from build123d import *

# Parameters (mm, degrees)
EXTRUDE_1_DEPTH     = 16
SKETCH_2_R          = 2.5
CUT_EXTRUDE_1_DEPTH = 9
SKETCH_3_R          = 4
CUT_EXTRUDE_2_DEPTH = 29


with BuildPart() as part:
    # 草图1 → 凸台-拉伸1 (new body)
    with BuildSketch(Plane.XY):
        Polygon((0, 0), (16, 0), (16, 8), (8, 8), (8, 40), (-8, 40), (-8, 8), (-16, 8), (-16, 0), align=None)
    extrude(amount=EXTRUDE_1_DEPTH)

    # 草图2 → 切除-拉伸1 (cut, through all)
    with BuildSketch(Plane(origin=(0, 8, 0), x_dir=(1, 0, 0), z_dir=(0, 1, 0))):
        with Locations((-12, -8)):
            Circle(SKETCH_2_R)
        with Locations((12, -8)):
            Circle(SKETCH_2_R)
    extrude(amount=-CUT_EXTRUDE_1_DEPTH, mode=Mode.SUBTRACT)

    # 草图3 → 切除-拉伸2 (cut)
    with BuildSketch(Plane.XY.offset(16)):
        with Locations((0, 31.77)):
            Circle(SKETCH_3_R)
    extrude(amount=-CUT_EXTRUDE_2_DEPTH, mode=Mode.SUBTRACT)


solid = part.part
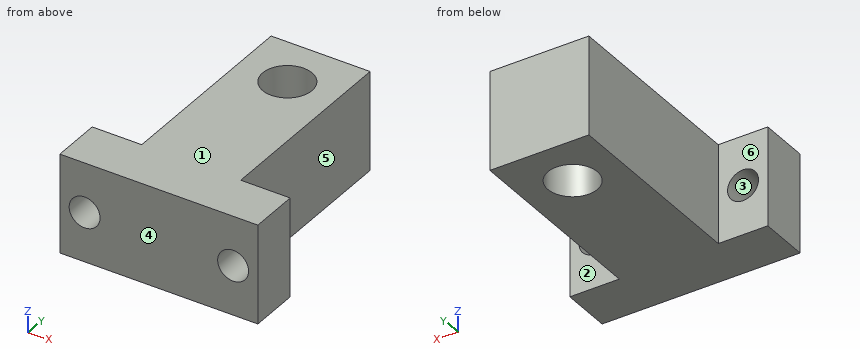
Geometry check sheet. Reference: the model listing, model coordinates, mm. Face numbers are marked on the shaded views. A direction names the side the tool comes from. Round coordinates to 2 decimals unless told otherwise and drop trailing zeros. Order: outer loops, then holes, each group sorted by start corner. A loop starts at its lowest first (then second) coordinate and runs counter-clockwise, first axis right, second up. Notation, with made-up numbers: M -14.75,-35 L 35.25,-35 A24 ccw 35.25,-10 Z; hole C 12,-8.5 d2. An arc over 180 degrees is marked long. Write each question's results on one line, items separated by ' | '. Start each with the question number.
1. Cross-section at D-D on z = 1. Record the boundary of the cut face in (x, y).
2. Set-up check for the marked faces 4, 5 and 6: record each of +Z, -Z, +X, -X, +Y, -Y from which the full face is reachable in a straight line by a thin tool's end or side.
3. Cross-section at A-A on z = 8. Record the boundary of the cut face in (x, y).
4. Material ranges on L1, parallel to X at y = 2.25, z = 8; L2, parallel to Y at x = 0, z = 5; L3, parallel to Z at x = -12, y = 3, recorded low to high. Write a range as from..to.
5. Cross-section at B-B on y = 31.77. Record the boundary of the cut face in (x, z), plus the area to 3 significant figures.
6. Cross-section at C-C on x = 0. Record the boundary of the cut face in (y, z).
7. Go/stop test with flat-tipped pins: P1, Ø6.5, axis at x = -12, z = 8, coming from the +Y side; P2, Ø1.5, axis at x = 0.5, y = 24, coming from the -Z side; P3, Ø1.5, axis at y = 9, z = 8.5, coming from the -X side; P4, Ø5, axis at y = 18, z = 10, coming from the +X side. Record where each tip stops, or that it passes through.
8. Draft check along Z on the marked faces 1, 2 and 3. Enter one of: pulls with the +Z half, pulls with the -Z half, needs draft (parallel to the pull), parting line crosses it, or undercut.
Resolved:
1) outline: M -16,0 L 16,0 L 16,8 L 8,8 L 8,40 L -8,40 L -8,8 L -16,8 Z; hole C 0,31.77 d8
2) face 4: +Z, -Z, +X, -X, -Y | face 5: +Z, -Z, +X, +Y | face 6: +Z, -Z, -X, +Y
3) outline: M -16,0 L -14.5,0 L -14.5,8 L -16,8 Z; M -9.5,0 L 9.5,0 L 9.5,8 L 8,8 L 8,40 L -8,40 L -8,8 L -9.5,8 Z; M 14.5,0 L 16,0 L 16,8 L 14.5,8 Z; hole C 0,31.77 d8
4) L1: -16..-14.5, -9.5..9.5, 14.5..16 | L2: 0..27.77, 35.77..40 | L3: 0..5.5, 10.5..16
5) outline: M -8,0 L -4,0 L -4,16 L -8,16 Z; M 4,0 L 8,0 L 8,16 L 4,16 Z | area: 128 mm2
6) outline: M 0,0 L 27.77,0 L 27.77,16 L 0,16 Z; M 35.77,0 L 40,0 L 40,16 L 35.77,16 Z
7) P1: y = 8 | P2: z = 0 | P3: x = -8 | P4: x = 8
8) face 1: pulls with the +Z half | face 2: needs draft | face 3: undercut
